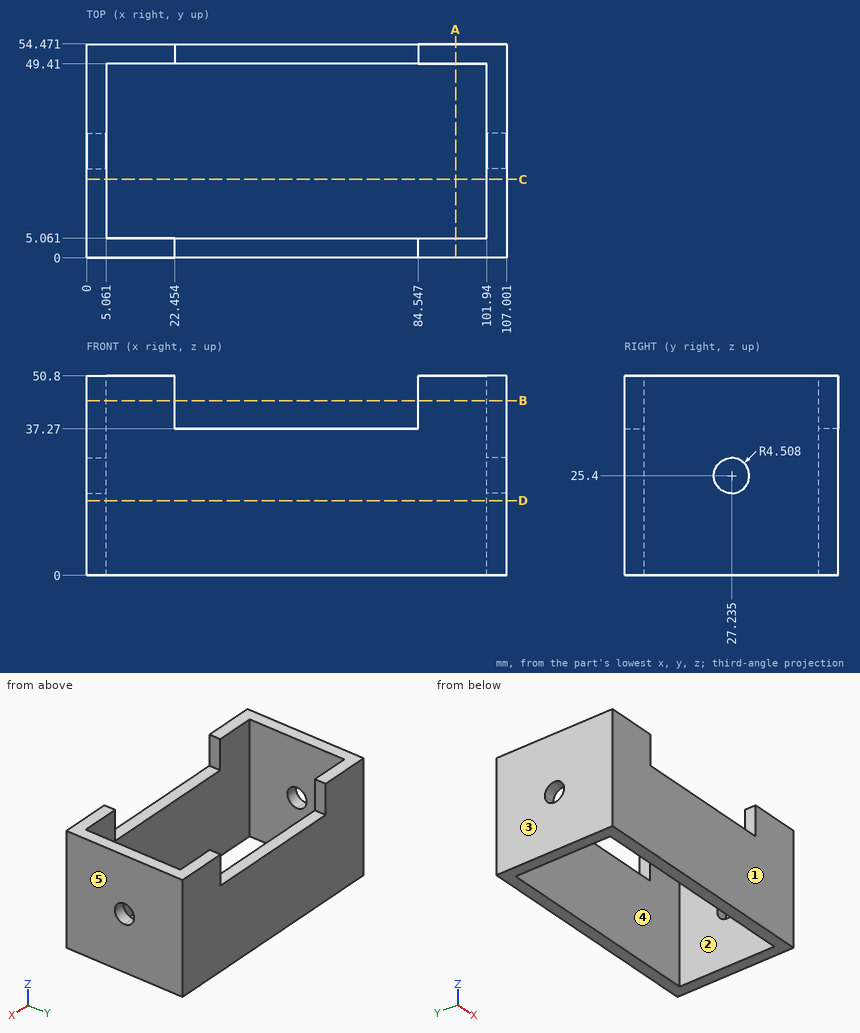
Print and shaded views of the part. All mm, measured from the part's lowest x, y and z. A direction names the side the tool comes from. Coordinates: 2 decimals unless noted, no trailing zeros. Order: outer loops, then holes, each group sorted by start corner. A loop starts at its lowest first (then second) coordinate and runs counter-clockwise, first axis right, second up. Notation, with made-up numbers: (52.5, -32) - (94.5, -32) arc R23 ccw to (94.5, -23) - close; hole circle Ø1 at (34.25, 2). An arc over 180 degrees is marked (long way). Return JSON: item names as keys, results as strings. Group by question number.
Item 1: Cut at C-C (y = 20). List the corners of the cut face in (x, z).
Item 2: Pull direction X, two halves, no side cores. Call the marked faces 1, 2 and 3: pulls with the +X half, pulls with the -X half, needs draft (parallel to the pull), parting line crosses it, or undercut.
Item 3: Pin check, flat tip, straight feed: pin 1 (1.5 mm diameter, centred on x = 52.5, y = 52, fed in from +Z). Stop position of the tip, or through.
Item 4: Cut at B-B (z = 44.5). List the corners of the cut face in (x, y) (1 decimal).
Item 5: Cut at D-D (z = 19). List the corners of the cut face in (x, y), plus the area to 3 significant figures.
Item 6: Cut at A-A (x = 94). List the corners of the cut face in (y, z).
Item 7: Drill centre lines: probe 1 along X at (y, z) = (19, 3.5); probe 2 along Y at (x, z) = (83, 21.5); probe 3 along Z at (x, y) = (33.5, 52.5). Where is each one in solid material? Low to high. Write a range as from..to.
Item 8: Which spindle directions (+Z, -Z, +X, -X, +Y, -Y) get a long thin tool onto all of the face, cutting with end or side? Do the marked faces 4 and 5. Say none if no direction does.
Check values:
{
 "1": {"outline": "(0, 0) - (5.06, 0) - (5.06, 50.8) - (0, 50.8) - close; (101.94, 0) - (107, 0) - (107, 50.8) - (101.94, 50.8) - close"},
 "2": {"face 1": "needs draft", "face 2": "undercut", "face 3": "pulls with the -X half"},
 "3": {"pin 1": "stops at z = 37.27"},
 "4": {"outline": "(0, 0) - (22.5, 0) - (22.5, 5.1) - (5.1, 5.1) - (5.1, 49.4) - (22.5, 49.4) - (22.5, 54.5) - (0, 54.5) - close; (84.5, 0) - (107, 0) - (107, 54.5) - (84.5, 54.5) - (84.5, 49.4) - (101.9, 49.4) - (101.9, 5.1) - (84.5, 5.1) - close"},
 "5": {"outline": "(0, 0) - (107, 0) - (107, 54.47) - (0, 54.47) - close; hole (5.06, 5.06) - (101.94, 5.06) - (101.94, 49.41) - (5.06, 49.41) - close", "area": "1,530 mm2"},
 "6": {"outline": "(0, 0) - (5.06, 0) - (5.06, 50.8) - (0, 50.8) - close; (49.41, 0) - (54.47, 0) - (54.47, 50.8) - (49.41, 50.8) - close"},
 "7": {"probe 1": "x = 0..5.06, 101.94..107", "probe 2": "y = 0..5.06, 49.41..54.47", "probe 3": "z = 0..37.27"},
 "8": {"face 4": "+Z, -Z", "face 5": "+Z, -Z, +X, +Y, -Y"}
}
